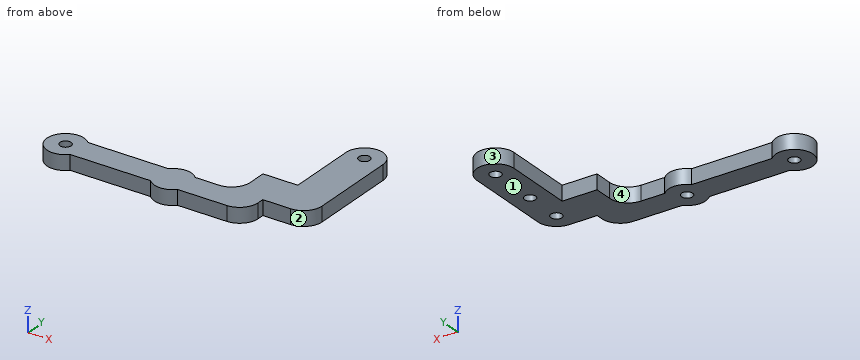
```python
from build123d import *

# Parameters (mm, degrees)
CROQUIS1_R              = 1.5
SALIENTE_EXTRUIR1_DEPTH = 4
SALIENTE_EXTRUIR2_START = -1
CROQUIS2_R              = 1.5
SALIENTE_EXTRUIR2_DEPTH = 1


with BuildPart() as part:
    # Croquis1 → Saliente-Extruir1 (new body)
    with BuildSketch(Plane.XY):
        with BuildLine():
            Line((51.875922813, -14.040123785), (59.395922813, -14.040123785))
            ThreePointArc((59.395922813, -14.040123785), (62.931456719, -12.575657691), (64.395922813, -9.040123785))
            Line((64.395922813, -9.040123785), (64.395922813, 14.699876215))
            ThreePointArc((64.395922813, 14.699876215), (59.395922813, 19.699876215), (54.395922813, 14.699876215))
            Line((54.395922813, 14.699876215), (54.395922813, -4.040123785))
            Line((54.395922813, -4.040123785), (44.995922813, -4.040123785))
            Line((44.995922813, -4.040123785), (44.995922813, -8.960123785))
            ThreePointArc((44.995922813, -8.960123785), (43.531456719, -12.495657691), (39.995922813, -13.960123785))
            Line((39.995922813, -13.960123785), (33.624476244, -13.960123785))
            ThreePointArc((33.624476244, -13.960123785), (29.995922813, -12.400123785), (26.367369382, -13.960123785))
            Line((26.367369382, -13.960123785), (4.684476244, -13.960123785))
            ThreePointArc((4.684476244, -13.960123785), (-3.944077187, -17.400123785), (4.684476244, -20.840123785))
            Line((4.684476244, -20.840123785), (26.367369382, -20.840123785))
            ThreePointArc((26.367369382, -20.840123785), (29.995922813, -22.400123785), (33.624476244, -20.840123785))
            Line((33.624476244, -20.840123785), (46.875922813, -20.840123785))
            ThreePointArc((46.875922813, -20.840123785), (50.411456719, -19.375657691), (51.875922813, -15.840123785))
            Line((51.875922813, -15.840123785), (51.875922813, -14.040123785))
        make_face()
        with Locations((59.395922813, -9.040123785)):
            Circle(CROQUIS1_R, mode=Mode.SUBTRACT)
        with Locations((59.395922813, 1.239876215)):
            Circle(CROQUIS1_R, mode=Mode.SUBTRACT)
        with Locations((59.395922813, 14.699876215)):
            Circle(CROQUIS1_R, mode=Mode.SUBTRACT)
        with Locations((29.995922813, -17.400123785)):
            Circle(CROQUIS1_R, mode=Mode.SUBTRACT)
        with Locations((1.055922813, -17.400123785)):
            Circle(CROQUIS1_R, mode=Mode.SUBTRACT)
    extrude(amount=SALIENTE_EXTRUIR1_DEPTH)

    # Croquis2 → Saliente-Extruir2 (add)
    with BuildSketch(Plane.XY.offset(4).offset(SALIENTE_EXTRUIR2_START)):
        with Locations((59.395922813, 1.239876215)):
            Circle(CROQUIS2_R)
        with Locations((59.395922813, -9.040123785)):
            Circle(CROQUIS2_R)
        with Locations((29.995922813, -17.400123785)):
            Circle(CROQUIS2_R)
    extrude(amount=SALIENTE_EXTRUIR2_DEPTH)


solid = part.part
```
The model under review builds one solid part; all positions refer to its coordinate system, in mm. Face numbers are marked on the shaded views. Round coordinates to 2 decimals unless told otherwise and drop trailing zeros. Write each loop counter-clockwise with the first axis right and the second up, starting at its lowest first coordinate (ties: lowest second). Pieces come first, ordered by that corner, then holes. Notation, with made-up numbers: M -14,18 L 31,18 A14 cw 31,41 Z; hole C 42.25,87 d3. An arc over 180 degrees is marked long. Use CSV: the item, a comma, the result in double quotes. Start each with the question number.
(1) Clearance check with flat-ended pins moving along their axes: P1, Ø1.2, axis at x = 15.5, z = 2, coming from the +Y side; P2, Ø2, axis at x = 55, z = 1.5, coming from the -Y side; P3, Ø0.9, axis at x = 30.5, y = -17, coming from the -Z side. State where each tip first meets the part, or that it passes through.
(2) We need section A-A, the plane z = 1. State the section outline as (x, y) points, then the cut area to 3 significant figures.
(3) We need section C-C, the plane x = 14. State the section outline as (y, z) points, then the cut area to 3 significant figures.
(4) For line 1 along Y through (x, z) = (1, 2.95); line 2 along X through (y, z) = (4, 2.55); line 3 along Y through (x, z) = (47, 1.7), list the stretches that pass through material, from the lowest coordinate up.
(5) We need section B-B, the plane y = 9. State the section outline as (x, z) points, then the cut area to 3 significant figures.
(6) The part is to be moulded in two halves that separate along X. For the marked faces 1, 2, 3 and 4, say which applies: +X half, -X half, draft (parallel to the pull), parting line (faces both ways), or undercut.
Findings:
1,P1,"y = -13.96"
1,P2,"y = -14.04"
1,P3,"z = 3"
2,outline,"M 4.68,-20.84 L 26.37,-20.84 A5 ccw 33.62,-20.84 L 46.88,-20.84 A5 ccw 51.88,-15.84 L 51.88,-14.04 L 59.4,-14.04 A5 ccw 64.4,-9.04 L 64.4,14.7 A5 ccw 54.4,14.7 L 54.4,-4.04 L 45,-4.04 L 45,-8.96 A5 cw 40,-13.96 L 33.62,-13.96 A5 ccw 26.37,-13.96 L 4.68,-13.96 A5 ccw long Z; hole C 1.06,-17.4 d3; hole C 30,-17.4 d3; hole C 59.4,-9.04 d3; hole C 59.4,1.24 d3; hole C 59.4,14.7 d3"
2,area,"792 mm^2"
3,outline,"M -20.84,0 L -13.96,0 L -13.96,4 L -20.84,4 Z"
3,area,"27.5 mm^2"
4,line 1,"-22.4 to -18.9, -15.9 to -12.4"
4,line 2,"54.4 to 64.4"
4,line 3,"-20.84 to -4.04"
5,outline,"M 54.4,0 L 64.4,0 L 64.4,4 L 54.4,4 Z"
5,area,"40.0 mm^2"
6,face 1,"draft"
6,face 2,"+X half"
6,face 3,"parting line"
6,face 4,"undercut"
